Here's how the part is built. I have some questions about the finished solid (model axes, mm). Face numbers are marked on the shaded views. A direction names the side the tool comes from. Coordinates: 2 decimals unless noted, no trailing zeros. Write each loop counter-clockwise with the first axis right and the second up, starting at its lowest first coordinate (ties: lowest second). Pieces come first, ordered by that corner, then holes.
(1) Which directions (+Z, -Z, +X, -X, +Y, -Y) give clear straight access to the entire face, cutting with the end or side of a thin tool? Please do the marked faces 4 and 5.
(2) For pin 1 Ø19 at (x, z) = (9.5, -19.5) entering from -Y; pin 2 Ø5 at (x, y) = (-40, -33) entering from -Z; pin 3 Ø12 at (x, z) = (-52.5, -12) entering from -Y, each with a flat end and sliding along its axis, tell me the tip position at first contact or that it passes through.
(3) Thinking about a two-plate mould opening in X: for the marked faces 1, 2 and 3, which applies, released by +X, released by -X, zero draft, split by the parting line, or undercut?
(4) Imagine slicing it at C-C, the plane z = -20. List the corners of the cut face in (x, y) for me.
(5) Imagine slicing it at D-D, the plane y = -57. List the corners of the cut face in (x, z) for me.
(6) Imagine slicing it at B-B, the plane y = -102. List the corners of the cut face in (x, z) for me (3 decimals), plus the area to 3 significant figures.
(7) Please list where these lines run through material, in increasing order: probe 1 along Y at (x, z) = (41.5, -1); probe 2 along Y at (x, z) = (-40, 15); probe 3 along Z at (x, y) = (-37.5, -59).
(8) Imagine slicing it at A-A, the plane z = 0. List the corners of the cut face in (x, y) for me.
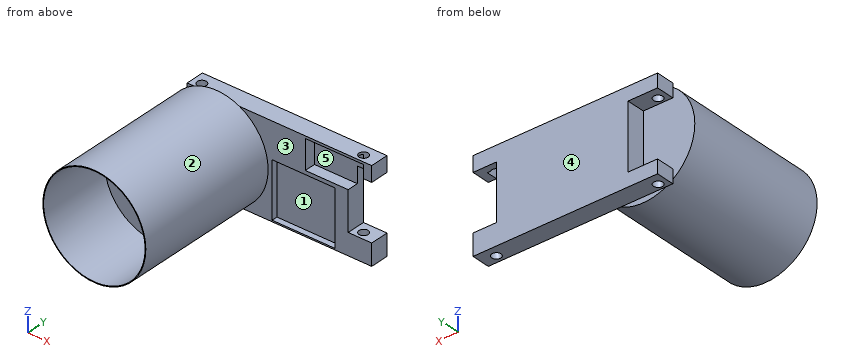
```python
from build123d import *

# Parameters (mm, degrees)
F0_W      = 127
F0_H      = 63.5
F1_DEPTH  = 12.7
F2_W      = 43.18
F2_H      = 38.1
F3_DEPTH  = 4
F4_W      = 39.997619
F4_H      = 20.153031
F5_DEPTH  = 7.62
F6_R      = 3.171763
F7_DEPTH  = 63.501
F8_R      = 3.175
F9_DEPTH  = 63.501
F10_W     = 32.382142
F10_H     = 38.156119
F11_DEPTH = 12.701
F12_W     = 40.605094
F12_H     = 44.755168
F13_DEPTH = 12.701
F14_R     = 35.422098
F15_DEPTH = 101.6
F16_R     = 34.925
F17_DEPTH = 50.8


with BuildPart() as f1:
    # F0 (on Front) → F1 (new body)
    with BuildSketch(Plane.XZ):
        Rectangle(F0_W, F0_H)
    extrude(amount=F1_DEPTH)

    # F2 (on face) → F3 (cut)
    with BuildSketch(Plane.XZ.offset(12.7)):
        with Locations((16.51, -11.7)):
            Rectangle(F2_W, F2_H)
    extrude(amount=-F3_DEPTH, mode=Mode.SUBTRACT)

    # F4 (on face) → F5 (cut)
    with BuildSketch(Plane.XZ.offset(12.7)):
        with Locations((37.80372, 20.028367)):
            Rectangle(F4_W, F4_H)
    extrude(amount=-F5_DEPTH, mode=Mode.SUBTRACT)

    # F6 (on face) → F7 (cut, through all)
    with BuildSketch(Plane(origin=(0, 0, -31.75), x_dir=(1, 0, 0), z_dir=(0, 0, -1))):
        with Locations((53.637695, 7.481154)):
            Circle(F6_R)
    extrude(amount=-F7_DEPTH, mode=Mode.SUBTRACT)

    # F8 (on face) → F9 (cut, through all)
    with BuildSketch(Plane(origin=(0, 0, -31.75), x_dir=(1, 0, 0), z_dir=(0, 0, -1))):
        with Locations((-57.188451, 8.090043)):
            Circle(F8_R)
    extrude(amount=-F9_DEPTH, mode=Mode.SUBTRACT)

    # F10 (on face) → F11 (cut, through all)
    with BuildSketch(Plane(origin=(0, 0, 0), x_dir=(-1, 0, 0), z_dir=(0, 1, 0))):
        with Locations((-63.5, 2.069221)):
            Rectangle(F10_W, F10_H)
    extrude(amount=-F11_DEPTH, mode=Mode.SUBTRACT)

    # F12 (on face) → F13 (cut, through all)
    with BuildSketch(Plane.XZ.offset(12.7)):
        with Locations((-63.5, 0)):
            Rectangle(F12_W, F12_H)
    extrude(amount=-F13_DEPTH, mode=Mode.SUBTRACT)

    # F14 (on face) → F15 (join)
    with BuildSketch(Plane.XZ.offset(12.7)):
        with Locations((-43.197453, 0)):
            Circle(F14_R)
    extrude(amount=F15_DEPTH)

    # F16 (on face) → F17 (cut)
    with BuildSketch(Plane.XZ.offset(114.3)):
        with Locations((-43.197453, 0)):
            Circle(F16_R)
    extrude(amount=-F17_DEPTH, mode=Mode.SUBTRACT)


solid = f1.part
```
Recorded:
1. face 4: +Z, -Z, +X, -X, +Y
1. face 5: -Y
2. pin 1: stops at y = -8.7
2. pin 2: stops at z = -35.42
2. pin 3: stops at y = -63.5
3. face 1: undercut
3. face 2: split by the parting line
3. face 3: zero draft
4. outline: (-72.43, -114.3) - (-71.83, -114.3) - (-71.83, -63.5) - (-14.57, -63.5) - (-14.57, -114.3) - (-13.96, -114.3) - (-13.96, -12.7) - (-5.08, -12.7) - (-5.08, -8.7) - (38.1, -8.7) - (38.1, -12.7) - (63.5, -12.7) - (63.5, 0) - (-43.2, 0) - (-43.2, -12.7) - (-72.43, -12.7) - close; hole circle Ø6.34 at (53.64, -7.48)
5. outline: circle Ø70.84 at (-43.2, 0)
6. outline: circle Ø70.844 at (-43.197, 0); hole circle Ø69.85 at (-43.197, 0)
6. area: 110 mm2
7. probe 1: y = -12.7 to 0
7. probe 2: y = -63.5 to 0
7. probe 3: z = -34.96 to 34.96
8. outline: (-78.62, -114.3) - (-78.12, -114.3) - (-78.12, -63.5) - (-8.27, -63.5) - (-8.27, -114.3) - (-7.78, -114.3) - (-7.78, -12.7) - (-5.08, -12.7) - (-5.08, -8.7) - (38.1, -8.7) - (38.1, -12.7) - (47.31, -12.7) - (47.31, 0) - (-43.2, 0) - (-43.2, -12.7) - (-78.62, -12.7) - close
